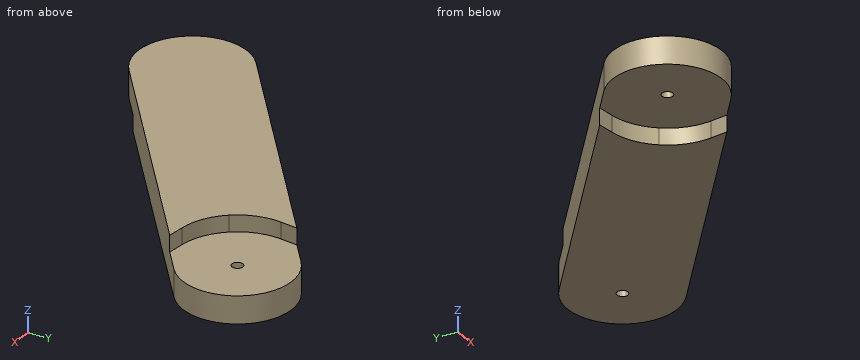
from build123d import *

# Parameters (mm, degrees)
BOSS_EXTRUDE1_DEPTH     = 20
CUT_EXTRUDE1_DEPTH      = 7.5
SKETCH3_R               = 2.5
CUT_EXTRUDE2_DEPTH      = 5
CUT_EXTRUDE3_START      = -7.5
SKETCH4_R               = 25
CUT_EXTRUDE3_DEPTH      = 7.5
CUT_EXTRUDE4_DEPTH      = 7.5
CUT_EXTRUDE5_DEPTH      = 187.21329098
CUT_EXTRUDE5_DEPTH_BACK = 7.5
SKETCH7_R               = 2.5
CUT_EXTRUDE6_DEPTH      = 186.557645323


with BuildPart() as part:
    # Sketch1 → Boss-Extrude1 (new body)
    with BuildSketch(Plane.XY):
        with BuildLine():
            Line((-15.358937815, 19.725694644), (102.995230052, 111.879321533))
            ThreePointArc((102.995230052, 111.879321533), (138.079862511, 107.512564703), (133.713105681, 72.427932244))
            Line((133.713105681, 72.427932244), (15.358937815, -19.725694644))
            ThreePointArc((15.358937815, -19.725694644), (-19.725694644, -15.358937815), (-15.358937815, 19.725694644))
        make_face()
    extrude(amount=BOSS_EXTRUDE1_DEPTH)

    # Sketch2 → Cut-Extrude1 (cut)
    with BuildSketch(Plane(origin=(0, 0, 0), x_dir=(-1, 0, 0), z_dir=(0, 0, -1))):
        with BuildLine():
            ThreePointArc((15.358937815, 19.725694644), (-19.725694644, 15.358937815), (-15.358937815, -19.725694644))
            ThreePointArc((-15.358937815, -19.725694644), (10.977853949, -22.460781881), (25, 0))
            ThreePointArc((25, 0), (22.460781881, 10.977853949), (15.358937815, 19.725694644))
        make_face()
    extrude(amount=-CUT_EXTRUDE1_DEPTH, mode=Mode.SUBTRACT)

    # Sketch3 → Cut-Extrude2 (cut)
    with BuildSketch(Plane(origin=(0, 0, 7.5), x_dir=(-1, 0, 0), z_dir=(0, 0, -1))):
        Circle(SKETCH3_R)
    extrude(amount=-CUT_EXTRUDE2_DEPTH, mode=Mode.SUBTRACT)

    # Sketch4 → Cut-Extrude3 (cut)
    with BuildSketch(Plane.XY.offset(20).offset(CUT_EXTRUDE3_START)):
        with Locations((118.354167866, 92.153626888)):
            Circle(SKETCH4_R)
    extrude(amount=CUT_EXTRUDE3_DEPTH, mode=Mode.SUBTRACT)

    # Sketch5 → Cut-Extrude4 (cut)
    with BuildSketch(Plane(origin=(0, 0, 0), x_dir=(-1, 0, 0), z_dir=(0, 0, -1))):
        with BuildLine():
            ThreePointArc((-3.396539703, 27.28943968), (-13.581209957, 23.912355302), (-21.698264109, 16.894831596))
            Line((-21.698264109, 16.894831596), (-19.725694644, 15.358937815))
            ThreePointArc((-19.725694644, 15.358937815), (-3.087763366, 24.808581527), (15.358937815, 19.725694644))
            Line((15.358937815, 19.725694644), (4.398653076, 28.259656807))
            Line((4.398653076, 28.259656807), (-3.396539703, 27.28943968))
        make_face()
        with BuildLine():
            Line((-27.28943968, -3.396539703), (-26.319222553, -11.191732482))
            Line((-26.319222553, -11.191732482), (-15.358937815, -19.725694644))
            ThreePointArc((-15.358937815, -19.725694644), (-24.808581527, -3.087763366), (-19.725694644, 15.358937815))
            Line((-19.725694644, 15.358937815), (-21.698264109, 16.894831596))
            ThreePointArc((-21.698264109, 16.894831596), (-26.511954246, 7.305222931), (-27.28943968, -3.396539703))
        make_face()
    extrude(amount=-CUT_EXTRUDE4_DEPTH, mode=Mode.SUBTRACT)

    # Sketch6 → Cut-Extrude5 (cut, two sides: drawn at the far end of the back side and taken through both)
    with BuildSketch(Plane.XY.offset(20).offset(-CUT_EXTRUDE5_DEPTH_BACK)):
        with BuildLine():
            Line((98.628473222, 76.794689074), (96.655903758, 75.258795292))
            ThreePointArc((96.655903758, 75.258795292), (104.77295791, 68.241271586), (114.957628164, 64.864187208))
            Line((114.957628164, 64.864187208), (122.752820943, 63.893970081))
            Line((122.752820943, 63.893970081), (133.713105681, 72.427932244))
            ThreePointArc((133.713105681, 72.427932244), (115.2664045, 67.345045361), (98.628473222, 76.794689074))
        make_face()
        with BuildLine():
            ThreePointArc((91.064728186, 95.550166591), (91.842213621, 84.848403957), (96.655903758, 75.258795292))
            Line((96.655903758, 75.258795292), (98.628473222, 76.794689074))
            ThreePointArc((98.628473222, 76.794689074), (93.545586339, 95.241390254), (102.995230052, 111.879321533))
            Line((102.995230052, 111.879321533), (92.034945313, 103.34535937))
            Line((92.034945313, 103.34535937), (91.064728186, 95.550166591))
        make_face()
    extrude(amount=CUT_EXTRUDE5_DEPTH + CUT_EXTRUDE5_DEPTH_BACK, mode=Mode.SUBTRACT)

    # Sketch7 → Cut-Extrude6 (cut, through all)
    with BuildSketch(Plane.XY.offset(12.5)):
        with Locations((118.354167866, 92.153626888)):
            Circle(SKETCH7_R)
    extrude(amount=-CUT_EXTRUDE6_DEPTH, mode=Mode.SUBTRACT)


solid = part.part
Here's how the part is built. I have some questions about the finished solid (model axes, mm). Give positions to 0.01 mm unless a question says otherwise; leave off trailing zeros. Loops run counter-clockwise (first coordinate to the right, second up) from the corner with the lowest first, then second, coordinate; pieces in that order, holes last. Notation, with made-up numbers: (20.25, -16.75) -> (69.25, -16.75) arc R32 ccw to (69.25, 14.25) -> close; hole circle Ø4 at (4, 72.5). An arc over 180 degrees is marked (long way). One line per item, written item: value.
Q1. If I drill on line 1 along Y through (x, z) = (0, 11.05); line 2 along Z through (x, y) = (106, 85); line 3 along Y through (x, z) = (101.5, 2.25), over which ranges is the centre line in solid material (lowest first)?
Answers follow:
line 1: -25 to -2.5, 2.5 to 31.68
line 2: 0 to 12.5
line 3: 47.35 to 110.72
Q2. I'm going to push flat-ended pins straight in: pin 1 Ø3 at (y, z) = (76, 7) entering from +X; pin 2 Ø4 at (x, y) = (0.5, -0.5) entering from -Z; pin 3 Ø1 at (x, z) = (41.5, 15) entering from -Y. Where does each tip first touch, or does it pass through?
Answers follow:
pin 1: x = 138.61
pin 2: z = 7.5
pin 3: y = 0.24
Q3. Suppose I cut it at D-D on y = 80. Please give me the cut outline in (x, z).
Answers follow:
outline: (62.05, 0) -> (140.2, 0) -> (140.2, 12.5) -> (93.69, 12.5) -> (93.69, 20) -> (62.05, 20) -> close
Q4. Suppose I cut it at A-A on z = 15.25. Please give me the cut outline in (x, y).
Answers follow:
outline: (-15.36, 19.73) arc R25 ccw to (15.36, -19.73) -> (122.75, 63.89) -> (114.96, 64.86) arc R27.5 cw to (91.06, 95.55) -> (92.03, 103.35) -> close
Q5. Suppose I cut it at C-C on x = 0. Please give me the cut outline in (y, z), then the cut area to 3 significant figures.
Answers follow:
outline: (-25, 7.5) -> (-2.5, 7.5) -> (-2.5, 12.5) -> (2.5, 12.5) -> (2.5, 7.5) -> (27.71, 7.5) -> (27.71, 0) -> (31.68, 0) -> (31.68, 20) -> (-25, 20) -> close
area: 713 mm^2
Q6. Suppose I cut it at B-B on y = -8. Please give me the cut outline in (x, z).
Answers follow:
outline: (-23.69, 7.5) -> (26.72, 7.5) -> (26.72, 0) -> (30.42, 0) -> (30.42, 20) -> (-23.69, 20) -> close
